from build123d import *

# Parameters (mm, degrees)
BOSS_EXTRUDE3_DEPTH = 3
SKETCH3_R           = 5
SKETCH2_R           = 2


with BuildPart() as part:
    # Sketch1 → Boss-Extrude3 (new body)
    with BuildSketch(Plane(origin=(0, 0, 0), x_dir=(1, 0, 0), z_dir=(0, 1, 0))):
        with BuildLine():
            Line((-78, 45.95), (78, 45.95))
            ThreePointArc((78, 45.95), (79.414213562, 45.364213562), (80, 43.95))
            Line((80, 43.95), (80, -43.95))
            ThreePointArc((80, -43.95), (79.414213562, -45.364213562), (78, -45.95))
            Line((78, -45.95), (-78, -45.95))
            ThreePointArc((-78, -45.95), (-79.414213562, -45.364213562), (-80, -43.95))
            Line((-80, -43.95), (-80, 43.95))
            ThreePointArc((-80, 43.95), (-79.414213562, 45.364213562), (-78, 45.95))
        make_face()
    extrude(amount=BOSS_EXTRUDE3_DEPTH)

    # Sketch3 → Loft1 section 0
    with BuildSketch(Plane(origin=(0, 8, 0), x_dir=(1, 0, 0), z_dir=(0, 1, 0))):
        with Locations((-75, 0)):
            Circle(SKETCH3_R)
    # Sketch2 → Loft1 section 1
    with BuildSketch(Plane(origin=(0, 3, 0), x_dir=(1, 0, 0), z_dir=(0, 1, 0))):
        with Locations((-75, 0)):
            Circle(SKETCH2_R)
    loft()


solid = part.part
Check sheet for the modelled part. Datum: model origin and axes. Units: mm. Give positions to 0.01 mm unless a question says otherwise; leave off trailing zeros. Write each loop counter-clockwise with the first axis right and the second up, starting at its lowest first coordinate (ties: lowest second). Pieces come first, ordered by that corner, then holes. Notation, with made-up numbers: M -12.75,84.5 L 7.25,84.5 A13 cw 7.25,107.5 Z; hole C 54,78.25 d11. An arc over 180 degrees is marked long. Use one line per item in the form item = value.
(1) Section check C-C on z = 22.5. Record the boundary of the cut face in (x, y).
Answer block:
outline = M -80,0 L 80,0 L 80,3 L -80,3 Z
(2) Material ranges on line 1 along Y through (x, z) = (32, -41); line 2 along X through (y, z) = (7, 2.5), recorded low to high.
Answer block:
line_1 = 0 to 3
line_2 = -78.62 to -71.38
(3) Section check D-D on x = -39. Record the boundary of the cut face in (y, z).
Answer block:
outline = M 0,-45.95 L 3,-45.95 L 3,45.95 L 0,45.95 Z
(4) Section check A-A on x = -75. Record the boundary of the cut face in (y, z), plus the area to 3 significant figures.
Answer block:
outline = M 0,-45.95 L 3,-45.95 L 3,-2 L 8,-5 L 8,5 L 3,2 L 3,45.95 L 0,45.95 Z
area = 311 mm2
(5) Draft check along Y on faces 1 (the flat face through (1, 0, -1)), 2 (the flat face through (-1, 1, -45.95)), 3 (the flat face through (-75, 8, 0)), 4 (the conical face through (-72.71, 3.8, 0.95)). Enter one of: pulls with the +Y half, pulls with the -Y half, needs draft (parallel to the pull), parting line crosses it, or undercut.
Answer block:
face_1 = pulls with the -Y half
face_2 = needs draft
face_3 = pulls with the +Y half
face_4 = undercut
(6) Section check B-B on y = 6.25. Record the boundary of the cut face in (x, z).
Answer block:
outline = C -75,0 d7.9
(7) Depth check by flat-ended pin: P1, Ø10, axis at x = -35, z = -28, coming from the +Y side. Enter the tip coordinate at first touch or a pass-through.
Answer block:
P1 = 3
